Verification items for the finished model (mm, model axes). Face numbers are marked on the shaded views. Give positions to 0.01 mm unless a question says otherwise; leave off trailing zeros. Loops run counter-clockwise (first coordinate to the right, second up) from the corner with the lowest first, then second, coordinate; pieces in that order, holes last. Notation, with made-up numbers: (35, 43.25) -> (56, 43.25) arc R17 cw to (56, 73.25) -> close; hole circle Ø8 at (-15.5, 4). An arc over 180 degrees is marked (long way). Answer in a Markdown table with one row per item. Add a question column.
Q1. Section check C-C on z = 2.3. Enter the section's corners in (x, y).
Q2. Release check for a two-part mould opening along X. For the marked faces 1, 2 and 3 record: pulls with the +X half, pulls with the -X half, needs draft (parallel to the pull), parting line crosses it, or undercut.
Q3. Material ranges on probe 1 along Y at (x, z) = (15, 2.8); probe 2 along X at (y, z) = (-1, 2.8); probe 3 along Y at (x, z) = (-1, 4.65), recorded low to high.
Q4. Section check B-B on y = 0. Enter the section's corners in (x, z).
Q5. Section check A-A on x = 15. Enter the section's corners in (y, z).
Q6. Gauge pin test, flat ends, axial feed: P1, Ø5, axis at x = -15, y = 0, coming from the +Z side; P2, Ø1.5, axis at y = 3, z = 3.5, coming from the -X side. Record the tip position at first contact, or that the pin passes through.
Q7. Section check D-D on x = -2. Enter the section's corners in (y, z), and give its area (3 significant figures).
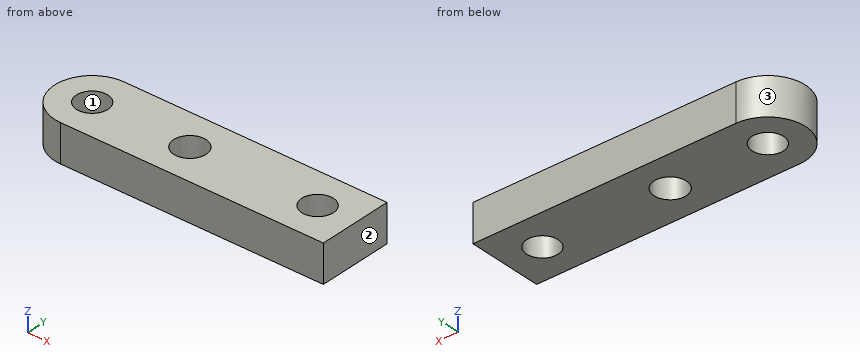
Autodesk Inventor part; units mm, degrees
ref_plane "YZ Plane" through (0, 0, 0) normal (1, 0, 0) x (0, 1, 0)
ref_plane "XZ Plane" through (0, 0, 0) normal (0, 1, 0) x (-1, 0, 0)
ref_plane "XY Plane" through (0, 0, 0) normal (0, 0, 1) x (1, 0, 0)
sketch "Sketch1" plane through (0, 0, 0) normal (0, 0, 1) x (1, 0, 0)
  line L0 (-15, 0) -> (15, 0) construction
  line L1 (-15, -5) -> (20, -5)
  line L2 (20, 5) -> (-15, 5)
  arc A0 (-15, 5) -> (-15, -5) centre (-15, 0) ccw
  arc A1 (15, -5) -> (15, 5) centre (15, 0) ccw construction
  circle A2 centre (-15, 0) radius 2.1
  circle A3 centre (15, 0) radius 2.1
  circle A4 centre (-2, 0) radius 2.15
  line L3 (20, 5) -> (20, -5)
  point P0 (0, 0)
  point P1 (0, 0)
  dimension "d0" = 5
  dimension "d1" = 4.2
  dimension "d2" = 4.2
  dimension "d3" = 30
  dimension "d6" = 4.3
  dimension "d7" = 17
extrude "Extrusion1" add sketch "Sketch1" along normal blind 5
properties part number "gate-pivot"
Taken from the geometry:
| question | item | result |
|---|---|---|
| 1 | outline | (-15, -5) -> (20, -5) -> (20, 5) -> (-15, 5) arc R5 ccw to start; hole circle Ø4.2 at (-15, 0); hole circle Ø4.3 at (-2, 0); hole circle Ø4.2 at (15, 0) |
| 2 | face 1 | undercut |
| 2 | face 2 | pulls with the +X half |
| 2 | face 3 | pulls with the -X half |
| 3 | probe 1 | y = -5 to -2.1, 2.1 to 5 |
| 3 | probe 2 | x = -19.9 to -16.85, -13.15 to -3.9, -0.1 to 13.15, 16.85 to 20 |
| 3 | probe 3 | y = -5 to -1.9, 1.9 to 5 |
| 4 | outline | (-20, 0) -> (-17.1, 0) -> (-17.1, 5) -> (-20, 5) -> close; (-12.9, 0) -> (-4.15, 0) -> (-4.15, 5) -> (-12.9, 5) -> close; (0.15, 0) -> (12.9, 0) -> (12.9, 5) -> (0.15, 5) -> close; (17.1, 0) -> (20, 0) -> (20, 5) -> (17.1, 5) -> close |
| 5 | outline | (-5, 0) -> (-2.1, 0) -> (-2.1, 5) -> (-5, 5) -> close; (2.1, 0) -> (5, 0) -> (5, 5) -> (2.1, 5) -> close |
| 6 | P1 | stops at z = 5 |
| 6 | P2 | stops at x = -19.47 |
| 7 | outline | (-5, 0) -> (-2.15, 0) -> (-2.15, 5) -> (-5, 5) -> close; (2.15, 0) -> (5, 0) -> (5, 5) -> (2.15, 5) -> close |
| 7 | area | 28.5 mm² |
